Here's the drawing with two shaded views (mm, measured from the low corner). I have some questions. A direction names the side the tool comes from. Give positions to 0.01 mm unless a question says otherwise; leave off trailing zeros. Write each loop counter-clockwise with the first axis right and the second up, starting at its lowest first coordinate (ties: lowest second). Pieces come first, ordered by that corner, then holes. Notation, with made-up numbers: (64, 6) - (114, 6) arc R28 ccw to (114, 39) - close; hole circle Ø8 at (-17.75, 89.5). An arc over 180 degrees is marked (long way). Use one line per item in the form item = value.
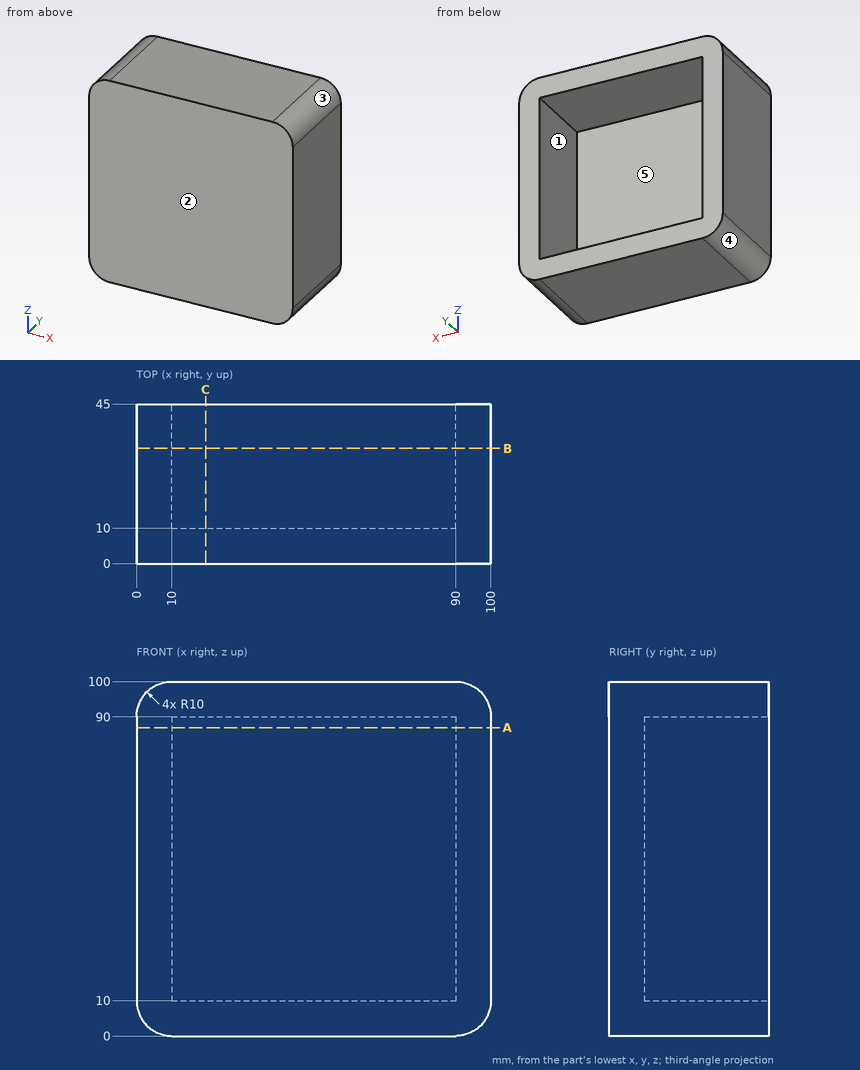
1. Imagine slicing it at B-B, the plane y = 32.5. List the corners of the cut face in (x, z) for me, and give its area (3 significant figures).
Response values:
outline = (0, 10) arc R10 ccw to (10, 0) - (90, 0) arc R10 ccw to (100, 10) - (100, 90) arc R10 ccw to (90, 100) - (10, 100) arc R10 ccw to (0, 90) - close; hole (10, 10) - (90, 10) - (90, 90) - (10, 90) - close
area = 3,510 mm²
2. Imagine slicing it at A-A, the plane z = 87. List the corners of the cut face in (x, y) for me, and give its area (3 significant figures).
Response values:
outline = (0, 0) - (100, 0) - (100, 45) - (90, 45) - (90, 10) - (10, 10) - (10, 45) - (0, 45) - close
area = 1,700 mm²
3. Imagine slicing it at C-C, the plane x = 19.5. List the corners of the cut face in (y, z) for me.
Response values:
outline = (0, 0) - (45, 0) - (45, 10) - (10, 10) - (10, 90) - (45, 90) - (45, 100) - (0, 100) - close
4. If I drill on line 1 (Z direction, x = 58, y = 34); line 2 (Y direction, x = 25.5, z = 68), over which ranges is the centre line in solid material (lowest first)? Write a range as from..to.
Response values:
line_1 = 0..10, 90..100
line_2 = 0..10
5. Which directions (+Z, -Z, +X, -X, +Y, -Y) give clear straight access to the entire face, cutting with the end or side of a thin tool? Please do the marked faces 4 and 5.
Response values:
face_4 = -Z, -X, +Y, -Y
face_5 = +Y
6. If we mould it in two halves opening along X, with no side actions, what happens to the marked faces 1, 2 and 3? For each: pulls with the +X half, pulls with the -X half, needs draft (parallel to the pull), parting line crosses it, or undercut.
Response values:
face_1 = undercut
face_2 = needs draft
face_3 = pulls with the +X half
7. For pin 1 (24 mm diameter, centred on x = 48, z = 47, fed in from +Y), with a flat end and sliding along its axis, tell me the tip position at first contact or that it passes through.
Response values:
pin_1 = 10
